Source: three-view drawing plus pictorial views. Frame: mm from the lowest corner of the part. Round coordinates to 2 decimals unless told otherwise and drop trailing zeros. Loops run counter-clockwise (first coordinate to the right, second up) from the corner with the lowest first, then second, coordinate; pieces in that order, holes last. Notation, with made-up numbers: M -14.5,-1 L -7.5,-1 A23 ccw -7.5,38 Z; hole C 36.25,34 d9. An arc over 180 degrees is marked long. Answer as a JSON object with one key per item and string values.
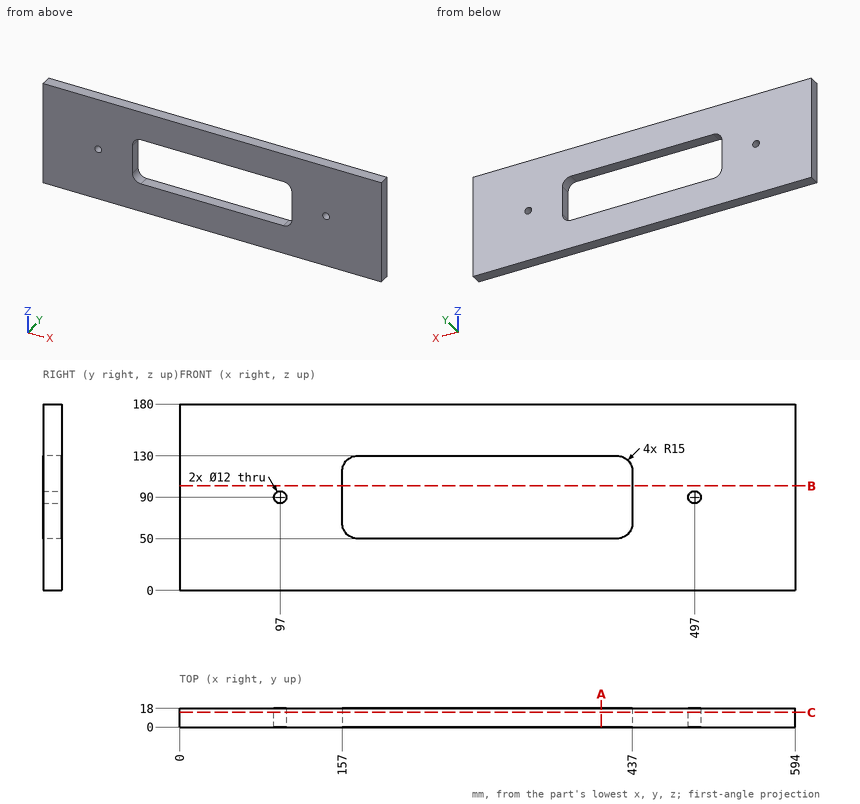
1) Line query: probe 1 along X at (y, z) = (10.75, 90); probe 2 along X at (y, z) = (7, 91); probe 3 along Z at (x, y) = (97, 11.75). Output: solid intervals per line, ascending.
Geometry results:
{"probe 1": "0 to 91, 103 to 157, 437 to 491, 503 to 594", "probe 2": "0 to 91.08, 102.92 to 157, 437 to 491.08, 502.92 to 594", "probe 3": "0 to 84, 96 to 180"}
2) Cut plane A-A on x = 407. Return the cut outline in (y, z), and give its area (3 significant figures).
Geometry results:
{"outline": "M 0,0 L 18,0 L 18,50 L 0,50 Z; M 0,130 L 18,130 L 18,180 L 0,180 Z", "area": "1,800 mm2"}
3) Cut plane C-C on y = 14.25. Return the cut outline in (x, z).
Geometry results:
{"outline": "M 0,0 L 594,0 L 594,180 L 0,180 Z; hole C 97,90 d12; hole M 157,65 A15 ccw 172,50 L 422,50 A15 ccw 437,65 L 437,115 A15 ccw 422,130 L 172,130 A15 ccw 157,115 Z; hole C 497,90 d12"}
4) Cut plane B-B on z = 101. Return the cut outline in (x, y), and give its area (3 significant figures).
Geometry results:
{"outline": "M 0,0 L 157,0 L 157,18 L 0,18 Z; M 437,0 L 594,0 L 594,18 L 437,18 Z", "area": "5,650 mm2"}
